Autodesk Fusion 360 part; units mm, degrees
box "BoxPrimitive1" add length 60 width 120 height 15 placed x (0, 0, -1) y (-1, 0, 0) z (0, 1, 0) at (120, 0, 0)
fillet "Fillet1" radius 20 1 edges at (0, 7.5, -60)
fillet "Fillet1" radius 20 1 edges at (120, 7.5, -60)
box "BoxPrimitive2" cut length 10.2 width 10.1 height -120 placed x (0, 1, 0) y (0, 0, 1) z (1, 0, 0) at (120, 2.4, -10.1)
box "BoxPrimitive3" cut length 30 width 80 height -60 placed x (0, 0, -1) y (-1, 0, 0) z (0, 1, 0) at (100, 15, -20)
fillet "Fillet2" radius 8 1 edges at (20, 7.5, -50)
fillet "Fillet2" radius 8 1 edges at (100, 7.5, -50)
fillet "Fillet2" radius 8 1 edges at (100, 7.5, -20)
fillet "Fillet2" radius 8 1 edges at (20, 7.5, -20)
cylinder "CylinderPrimitive1" cut diameter 3.2 height -15 placed x (1, 0, 0) y (0, 0, -1) z (0, 1, 0) at (60, 15, -5)
cylinder "CylinderPrimitive2" cut diameter 3.2 height -15 placed x (1, 0, 0) y (0, 0, -1) z (0, 1, 0) at (20, 15, -5)
cylinder "CylinderPrimitive3" cut diameter 3.2 height -15 placed x (1, 0, 0) y (0, 0, -1) z (0, 1, 0) at (100, 15, -5)
fillet "Fillet3" radius 3 8 edges at (60, 15, -50) (22.3431, 15, -47.6569) (20, 15, -35) (22.3431, 15, -22.3431) (60, 15, -20) (97.6569, 15, -22.3431) (100, 15, -35) (97.6569, 15, -47.6569)
fillet "Fillet3" radius 3 8 edges at (97.6569, 0, -47.6569) (60, 0, -50) (22.3431, 0, -47.6569) (20, 0, -35) (22.3431, 0, -22.3431) (60, 0, -20) (97.6569, 0, -22.3431) (100, 0, -35)
fillet "Fillet4" radius 1 1 edges at (120, 13.8, 0)
fillet "Fillet4" radius 1 1 edges at (120, 1.2, 0)
fillet "Fillet4" radius 1 1 edges at (0, 13.8, 0)
fillet "Fillet4" radius 1 1 edges at (0, 1.2, 0)
Input: part model. Units: mm. Frame: model coordinates. A direction names the side the tool comes from. Give positions to 0.01 mm unless a question says otherwise; leave off trailing zeros. Order: outer loops, then holes, each group sorted by start corner. A loop starts at its lowest first (then second) coordinate and runs counter-clockwise, first axis right, second up.
1. Cut plane D-D (y = 5). Return loops of the section in (x, z), and give its area (3 significant figures).
Computed:
outline: (0, -40) arc R20 ccw to (20, -60) - (100, -60) arc R20 ccw to (120, -40) - (120, -10.1) - (0, -10.1) - close; hole (20, -42) arc R8 ccw to (28, -50) - (92, -50) arc R8 ccw to (100, -42) - (100, -28) arc R8 ccw to (92, -20) - (28, -20) arc R8 ccw to (20, -28) - close
area: 3,470 mm2
2. Line query: probe 1 along X at (y, z) = (13.7, -5); probe 2 along Y at (x, z) = (50.5, -9); probe 3 along Z at (x, y) = (100, 14.05). Output: solid intervals per line, ascending.
Computed:
probe 1: x = 0 to 18.4, 21.6 to 58.4, 61.6 to 98.4, 101.6 to 120
probe 2: y = 0 to 2.4, 12.6 to 15
probe 3: z = -60 to -45.69, -24.31 to -6.6, -3.4 to 0
3. Pin query (flat end, axial travel): pin 1 Ø3 at (x, y) = (54.5, 8) entering from +Z; pin 2 Ø5 at (y, z) = (12, -48.5) entering from +X. Return the tip coordinate at first contact, or that it passes through.
Computed:
pin 1: stops at z = -10.1
pin 2: stops at x = 119.08
4. Cut plane B-B (x = 78). Return loops of the section in (y, z).
Computed:
outline: (0, -60) - (15, -60) - (15, -53) arc R3 ccw to (12, -50) - (3, -50) arc R3 ccw to (0, -53) - close; (0, -17) arc R3 ccw to (3, -20) - (12, -20) arc R3 ccw to (15, -17) - (15, 0) - (12.6, 0) - (12.6, -10.1) - (2.4, -10.1) - (2.4, 0) - (0, 0) - close
5. Draft query along Z for faces 5 (the face through (22.281, 7.563, -22.406)), 6 (the face through (59, 8, -10.1)), 7 (the face through (61, 7, -60)), 8 (the face through (59, 15, -16)). Return one class per face: released by +Z, released by -Z, zero draft, split by the parting line, or undercut.
Computed:
face 5: undercut
face 6: released by +Z
face 7: released by -Z
face 8: zero draft
6. Cut plane A-A (z = -5). State how many separate pieces and enclosed holes the cut face has, and give its area (3 significant figures).
Computed:
separate pieces: 8
enclosed holes: 0
area: 530 mm2
7. Set-up query: faces 1 (the face through (59.55, 14.1, -50.86)), 2 (the face through (59, 2.4, -7)), 3 (the face through (60.45, 0.86, -19.1)), 4 (the face through (97.594, 7.563, -22.281)). Return all of +Z, -Z, +X, -X, +Y, -Y with unobstructed straight access to the full face (end or side cutting, diameter ignored); none if empty.
Computed:
face 1: +Y
face 2: +Z, +X, -X
face 3: -Y
face 4: +Y, -Y
8. Cut plane C-C (x = 60). Return loops of the section in (y, z), and give its area (3 significant figures).
Computed:
outline: (0, -60) - (15, -60) - (15, -53) arc R3 ccw to (12, -50) - (3, -50) arc R3 ccw to (0, -53) - close; (0, -17) arc R3 ccw to (3, -20) - (12, -20) arc R3 ccw to (15, -17) - (15, -6.6) - (12.6, -6.6) - (12.6, -10.1) - (2.4, -10.1) - (2.4, -6.6) - (0, -6.6) - close; (0, -3.4) - (2.4, -3.4) - (2.4, 0) - (0, 0) - close; (12.6, -3.4) - (15, -3.4) - (15, 0) - (12.6, 0) - close
area: 324 mm2
